Autodesk Inventor part; units mm, degrees
ref_plane "YZ Plane" through (0, 0, 0) normal (1, 0, 0) x (0, 1, 0)
ref_plane "XZ Plane" through (0, 0, 0) normal (0, 1, 0) x (-1, 0, 0)
ref_plane "XY Plane" through (0, 0, 0) normal (0, 0, 1) x (1, 0, 0)
sketch "Sketch1" plane through (0, 0, 0) normal (0, 1, 0) x (-1, 0, 0)
  line L0 (0, 0) -> (3.15, 0)
  line L1 (3.15, 0) -> (3.15, -20)
  line L2 (3.15, -20) -> (0, -20)
  line L3 (0, -20) -> (0, 0)
  line L4 (0, 0) -> (20, 0)
  line L5 (20, 0) -> (20, -3.15)
  line L6 (20, -3.15) -> (0, -3.15)
  line L7 (0, -3.15) -> (0, 0)
  line L8 (-1.5, 1.5) -> (4.65, 1.5)
  line L9 (4.65, 1.5) -> (4.65, -21.5)
  line L10 (4.65, -21.5) -> (-1.5, -21.5)
  line L11 (-1.5, -21.5) -> (-1.5, 1.5)
  line L12 (21.5, 1.5) -> (-1.5, 1.5)
  line L13 (-1.5, 1.5) -> (-1.5, -4.65)
  line L14 (-1.5, -4.65) -> (21.5, -4.65)
  line L15 (21.5, -4.65) -> (21.5, 1.5)
  line L16 (3.15, -20) -> (3.15, -21.5)
  line L17 (0, -20) -> (0, -21.5)
  line L18 (20, 0) -> (21.5, 0)
  line L19 (20, -3.15) -> (21.5, -3.15)
  line L20 (0, 0) -> (87.6, 0)
  line L21 (87.6, 0) -> (87.6, -3.15)
  line L22 (87.6, -3.15) -> (0, -3.15)
  line L23 (0, -3.15) -> (0, 0)
  line L24 (87.6, 0) -> (89.1, 0)
  line L25 (89.1, 0) -> (89.1, -21.5)
  line L26 (89.1, -21.5) -> (87.6, -21.5)
  line L27 (87.6, -21.5) -> (87.6, 0)
  line L28 (89.1, 0) -> (69.1, 0)
  line L29 (69.1, 0) -> (69.1, 1.5)
  line L30 (69.1, 1.5) -> (89.1, 1.5)
  line L31 (89.1, 1.5) -> (89.1, 0)
  line L32 (87.6, -3.15) -> (84.45, -3.15)
  line L33 (84.45, -3.15) -> (84.45, -21.5)
  line L34 (84.45, -21.5) -> (87.6, -21.5)
  line L35 (87.6, -21.5) -> (87.6, -3.15)
  line L36 (84.45, -3.15) -> (82.95, -3.15)
  line L37 (82.95, -3.15) -> (82.95, -21.5)
  line L38 (82.95, -21.5) -> (84.45, -21.5)
  line L39 (84.45, -21.5) -> (84.45, -3.15)
  line L40 (82.95, -3.15) -> (69.1, -3.15)
  line L41 (69.1, -3.15) -> (69.1, -4.65)
  line L42 (69.1, -4.65) -> (82.95, -4.65)
  line L43 (82.95, -4.65) -> (82.95, -3.15)
  line L44 (69.1, -4.65) -> (21.5, -4.65)
  line L45 (21.5, -4.65) -> (21.5, -3.15)
  line L46 (21.5, -3.15) -> (69.1, -3.15)
  line L47 (69.1, -3.15) -> (69.1, -4.65)
  line L48 (69.1, 1.5) -> (21.5, 1.5)
  line L49 (21.5, 1.5) -> (21.5, 0)
  line L50 (21.5, 0) -> (69.1, 0)
  line L51 (69.1, 0) -> (69.1, 1.5)
  point P0 (3.15, -3.15)
  point P1 (4.65, -4.65)
  point P2 (4.65, 1.5)
  point P3 (69.1, 0)
  point P4 (84.45, -3.15)
  point P5 (69.1, -3.15)
  point P6 (21.5, -4.65)
  point P7 (21.5, -3.15)
  dimension "d0" = 3.15
  dimension "d1" = 3.15
  dimension "d2" = 20
  dimension "d3" = 20
  dimension "d4" = 1.5
  dimension "d5" = 1.5
  dimension "d16" = 87.6
  dimension "d17" = 0
  dimension "d18" = 0
  dimension "d19" = 20
  dimension "d20" = 1.5
  dimension "d21" = 3.15
  dimension "d22" = 0
  dimension "d23" = 0
  dimension "d24" = 0
  dimension "d25" = 0
  dimension "d26" = 1.5
  dimension "d27" = 1.5
extrude "Extrusion1" add sketch "Sketch1" along normal blind 5 contours L3 L14 L11 L8 L9 L4 L0 | L6 L9 L14 L1 | L9 L12 L15 L18 L4 | L3 L17 L10 L11 L14 | L14 L9 L10 L16 L1 | L6 L19 L15 L14 L9 | L15 L48 L29 L20 | L15 L22 L41 L44 | L29 L30 L31 L24 L20 | L41 L22 L37 L42 | L24 L25 L26 L27 L21 | L37 L22 L33 L38
sketch "Sketch2" plane through (0, 5, 0) normal (0, 1, 0) x (1, 0, 0)
  line L0 (-3.15, 3.15) -> (-3.15, 21.5)
  line L1 (-3.15, 21.5) -> (-4.65, 21.5)
  line L2 (-4.65, 21.5) -> (-4.65, 4.65)
  line L3 (1.5, -1.5) -> (1.5, 21.5)
  line L4 (1.5, 21.5) -> (0, 21.5)
  line L5 (0, 21.5) -> (0, 0)
  line L6 (0, 0) -> (-21.5, 0)
  line L7 (-21.5, 0) -> (-21.5, 3)
  line L8 (-3.15, 3.15) -> (-3.15, 21.5)
  line L9 (-3.15, 21.5) -> (0, 21.5)
  line L10 (-89.1, 21.5) -> (-89.1, -1.5)
  line L11 (-82.95, 4.65) -> (-82.95, 21.5)
  line L12 (-89.1, -1.5) -> (-68.78, -1.5)
  line L13 (-68.78, 4.5) -> (-82.95, 4.5)
  line L14 (-87.6, 21.5) -> (-89.1, 21.5)
  line L15 (-89.1, 21.5) -> (-82.95, 21.5)
  line L16 (-82.95, 21.5) -> (-82.95, -1.5)
  line L17 (-82.95, -1.5) -> (-89.1, -1.5)
  line L18 (-89.1, -1.5) -> (-89.1, 21.5)
  line L19 (-68.78, -1.5) -> (-82.95, -1.5)
  line L20 (-82.95, -1.5) -> (-82.95, 4.65)
  line L21 (-82.95, 4.65) -> (-68.78, 4.65)
  line L22 (-68.78, 4.65) -> (-68.78, -1.5)
  line L23 (0, 0) -> (-87.6, 0)
  line L24 (-87.6, 0) -> (-87.6, 21.5)
  line L25 (-87.6, 21.5) -> (-89.1, 21.5)
  line L26 (-89.1, 21.5) -> (-89.1, -1.5)
  line L27 (-89.1, -1.5) -> (1.5, -1.5)
  line L28 (-84.45, 3.15) -> (-3.15, 3.15)
  line L29 (-4.65, 4.65) -> (-82.95, 4.65)
  line L30 (-82.95, 4.65) -> (-82.95, 21.5)
  line L31 (-82.95, 21.5) -> (-84.45, 21.5)
  line L32 (-84.45, 21.5) -> (-84.45, 3.15)
  point P0 (-82.95, 4.65)
  point P1 (-68.78, 4.65)
  dimension "d31" = 0
extrude "Extrusion2" add sketch "Sketch2" along normal blind 2
sketch "Sketch3" plane through (0, 0, 0) normal (0, -1, 0) x (1, 0, 0)
  line L0 (-4.65, -21.5) -> (-4.65, -4.65)
  line L1 (-3.15, -21.5) -> (-4.65, -21.5)
  line L2 (-3.15, -3.15) -> (-3.15, -21.5)
  line L3 (0, -21.5) -> (0, 0)
  line L4 (1.5, -21.5) -> (0, -21.5)
  line L5 (1.5, 1.5) -> (1.5, -21.5)
  line L6 (-21.5, -3) -> (-3.15, -3)
  line L7 (-4.65, -21.5) -> (-4.65, -4.65)
  line L8 (-3.15, -3.15) -> (-4.65, -3.15)
  line L9 (-4.65, -3.15) -> (-4.65, -13.15)
  line L10 (-4.65, -13.15) -> (-3.15, -13.15)
  line L11 (-3.15, -13.15) -> (-3.15, -3.15)
  line L12 (-3.15, -3.15) -> (-3.15, -21.5)
  line L13 (-3.15, -3.15) -> (-13.15, -3.15)
  line L14 (-13.15, -3.15) -> (-13.15, -4.65)
  line L15 (-13.15, -4.65) -> (-3.15, -4.65)
  line L16 (-3.15, -4.65) -> (-3.15, -3.15)
  line L17 (-21.5, 1.5) -> (1.5, 1.5)
  line L18 (0, -21.5) -> (0, 0)
  line L19 (1.5, 1.5) -> (0, 1.5)
  line L20 (0, 1.5) -> (0, -13.15)
  line L21 (0, -13.15) -> (1.5, -13.15)
  line L22 (1.5, -13.15) -> (1.5, 1.5)
  line L23 (1.5, 1.5) -> (-13.15, 1.5)
  line L24 (-13.15, 1.5) -> (-13.15, 0)
  line L25 (-13.15, 0) -> (1.5, 0)
  line L26 (1.5, 0) -> (1.5, 1.5)
  line L27 (-89.1, -21.5) -> (-89.1, 1.5)
  line L28 (0, 0) -> (-87.6, 0)
  line L29 (-89.1, 1.5) -> (-74.45, 1.5)
  line L30 (-74.45, 1.5) -> (-74.45, 0)
  line L31 (-74.45, 0) -> (-89.1, 0)
  line L32 (-89.1, 0) -> (-89.1, 1.5)
  line L33 (-89.1, 1.5) -> (-68.78, 1.5)
  line L34 (-89.1, 1.5) -> (-87.6, 1.5)
  line L35 (-87.6, 1.5) -> (-87.6, -13.15)
  line L36 (-87.6, -13.15) -> (-89.1, -13.15)
  line L37 (-89.1, -13.15) -> (-89.1, 1.5)
  line L38 (-84.45, -21.5) -> (-84.45, -3.15)
  line L39 (-74.45, -3.15) -> (-84.45, -3.15)
  line L40 (-84.45, -3.15) -> (-84.45, -4.65)
  line L41 (-84.45, -4.65) -> (-74.45, -4.65)
  line L42 (-74.45, -4.65) -> (-74.45, -3.15)
  line L43 (-84.45, -3.15) -> (-3.15, -3.15)
  line L44 (-82.95, -4.65) -> (-82.95, -21.5)
  line L45 (-84.45, -3.15) -> (-82.95, -3.15)
  line L46 (-82.95, -3.15) -> (-82.95, -13.075)
  line L47 (-82.95, -13.075) -> (-84.45, -13.075)
  line L48 (-84.45, -13.075) -> (-84.45, -3.15)
  line L49 (0, 0) -> (-87.6, 0)
  line L50 (-89.1, 1.5) -> (1.5, 1.5)
  line L51 (-89.1, -21.5) -> (-89.1, 1.5)
  line L52 (-87.6, -21.5) -> (-89.1, -21.5)
  line L53 (-87.6, 0) -> (-87.6, -21.5)
  line L54 (-84.45, -3.15) -> (-3.15, -3.15)
  line L55 (-84.45, -21.5) -> (-84.45, -3.15)
  line L56 (-82.95, -21.5) -> (-84.45, -21.5)
  line L57 (-82.95, -4.65) -> (-82.95, -21.5)
  line L58 (-4.65, -4.65) -> (-82.95, -4.65)
  point P0 (-3.15, -13.15)
  point P1 (-68.78, 0)
  point P2 (-68.78, -3)
  point P3 (1.5, 0)
  point P4 (-3.15, -4.65)
  point P5 (-4.65, -4.65)
  point P6 (-13, -3)
  point P7 (-4.65, -4.65)
  dimension "d10" = 10
  dimension "d11" = 10
  dimension "d12" = 14.65
  dimension "d13" = 14.65
  dimension "d28" = 14.65
  dimension "d29" = 14.65
  dimension "d30" = 10
  dimension "d32" = 0
  dimension "d33" = 0
extrude "Extrusion3" add sketch "Sketch3" along normal blind 5 contours L0 L15 L2 L10 | L15 L14 L13 L9 | L9 L8 L2 L15 | L41 L46 L39 L42 | L44 L47 L38 L41 | L41 L38 L39 L46 | L3 L25 L5 L21 | L25 L24 L17 L20 | L20 L17 L5 L25 | L28 L35 L29 L30 | L35 L36 L27 L31 | L31 L27 L29 L35
properties part number "Glass ConnectorV2"
Part model, mm, in its own coordinate system. A direction names the side the tool comes from. Give positions to 0.01 mm unless a question says otherwise; leave off trailing zeros. Order: outer loops, then holes, each group sorted by start corner. A loop starts at its lowest first (then second) coordinate and runs counter-clockwise, first axis right, second up. Notation, with made-up numbers: (-35.5, 61.25) - (19.5, 61.25) arc R19 ccw to (19.5, 84.25) - close; hole circle Ø10 at (-21, -21.75). An arc over 180 degrees is marked (long way). One line per question, with ' | ' between items.
1. Band-saw the part on B-B on z = -9.25. List the corners of the cut face in (x, y), then the cut area to 3 significant figures.
Filled in:
outline: (-89.1, -5) - (-87.6, -5) - (-87.6, 5) - (-84.45, 5) - (-84.45, -5) - (-82.95, -5) - (-82.95, 7) - (-89.1, 7) - close; (-4.65, -5) - (-3.15, -5) - (-3.15, 5) - (0, 5) - (0, -5) - (1.5, -5) - (1.5, 7) - (-4.65, 7) - close | area: 84.6 mm²
2. Band-saw the part on D-D on y = -3.75. List the corners of the cut face in (x, z) (3 decimals), then the cut area to 3 significant figures.
Filled in:
outline: (-89.1, -13.15) - (-87.6, -13.15) - (-87.6, 0) - (-74.45, 0) - (-74.45, 1.5) - (-89.1, 1.5) - close; (-84.45, -13.075) - (-82.95, -13.075) - (-82.95, -4.65) - (-74.45, -4.65) - (-74.45, -3.15) - (-84.45, -3.15) - close; (-13.15, -4.65) - (-4.65, -4.65) - (-4.65, -13.15) - (-3.15, -13.15) - (-3.15, -3.15) - (-13.15, -3.15) - close; (-13.15, 0) - (0, 0) - (0, -13.15) - (1.5, -13.15) - (1.5, 1.5) - (-13.15, 1.5) - close | area: 139 mm²
3. Band-saw the part on A-A on y = 4. List the corners of the cut face in (x, z), then the cut area to 3 significant figures.
Filled in:
outline: (-89.1, -21.5) - (-87.6, -21.5) - (-87.6, 0) - (0, 0) - (0, -21.5) - (1.5, -21.5) - (1.5, 1.5) - (-89.1, 1.5) - close; (-84.45, -21.5) - (-82.95, -21.5) - (-82.95, -4.65) - (-4.65, -4.65) - (-4.65, -21.5) - (-3.15, -21.5) - (-3.15, -3.15) - (-84.45, -3.15) - close | area: 373 mm²
4. Drop flat-ended pins along their axis: P1, Ø1.6, axis at x = 0.5, y = -2, coming from the -Z side; P2, Ø1.5, axis at x = -37.5, y = 3, coming from the -Z side; P3, Ø8, axis at x = -8, z = -17.5, coming from the -Y side; P4, Ø6.5, axis at x = -37, z = -8.5, coming from the -Y side. Give the stop position or say it passes through.
Filled in:
P1: z = -13.15 | P2: z = -4.65 | P3: y = 0 | P4: through
5. Band-saw the part on C-C on x = -9. List the corners of the cut face in (y, z).
Filled in:
outline: (-5, -4.65) - (7, -4.65) - (7, 1.5) - (-5, 1.5) - (-5, 0) - (5, 0) - (5, -3.15) - (-5, -3.15) - close
6. Which spindle directions (+Z, -Z, +X, -X, +Y, -Y) get a long thin tool onto all of the face, cutting with end or side? Do faces 4 (the face through (-74.45, -2, 1)), 5 (the face through (-88, -2, -13.15)), 6 (the face through (-3.15, 1, -10)), 7 (the face through (-43, 2, 0)), 8 (the face through (-82.95, 2, -11)). Say none if no direction does.
Filled in:
face 4: +Z, -Z, -Y | face 5: -Z, +X, -X, -Y | face 6: -Z, -Y | face 7: -Y | face 8: -Z, +Y, -Y
7. Drill centre lines: probe 1 along X at (y, z) = (4.25, -17); probe 2 along X at (y, z) = (-1.25, -3.5); probe 3 along Z at (x, y) = (-39, 0.25). Where is each one in solid material? Low to high.
Filled in:
probe 1: -89.1 to -87.6, -84.45 to -82.95, -4.65 to -3.15, 0 to 1.5 | probe 2: -89.1 to -87.6, -84.45 to -74.45, -13.15 to -3.15, 0 to 1.5 | probe 3: -4.65 to -3.15, 0 to 1.5
8. Pull direction X, two halves, no side cores. Call faces 1 (the face through (-89.1, 1, -7)), 2 (the face through (-88, 0, -17)), 3 (the face through (-43, 2, -4.65)): +X half, -X half, draft (parallel to the pull), parting line (faces both ways), or undercut.
Filled in:
face 1: -X half | face 2: draft | face 3: undercut
